```python
from build123d import *

# Parameters (mm, degrees)
F1_DEPTH = 10
F2_DEPTH = 12
F3_SIZE  = 5
F4_SIZE  = 1.99999
F5_R     = 10
F6_DEPTH = 5
F7_R     = 4.99999
F9_DEPTH = 3


# Not quite as in the source:
# - a fillet or chamfer is up to 0.001 mm smaller than in the source, because OpenCascade refuses the exact size


with BuildPart() as f1:
    # F0 (on Right) → F1 (new body)
    with BuildSketch(Plane.YZ):
        with BuildLine():
            Line((15, 5), (27.0370116692, 13))
            ThreePointArc((27.0370116692, 13), (21.2132034356, 21.2132034356), (13, 27.0370116692))
            Line((13, 27.0370116692), (5, 15))
            Line((5, 15), (0, 15))
            Line((0, 15), (-5, 15))
            Line((-5, 15), (-13, 27.0370116692))
            ThreePointArc((-13, 27.0370116692), (-21.2132034356, 21.2132034356), (-27.0370116692, 13))
            Line((-27.0370116692, 13), (-15, 5))
            Line((-15, 5), (-15, 0))
            Line((-15, 0), (-15, -5))
            Line((-15, -5), (-27.0370116692, -13))
            ThreePointArc((-27.0370116692, -13), (-21.2132034356, -21.2132034356), (-13, -27.0370116692))
            Line((-13, -27.0370116692), (-5, -15))
            Line((-5, -15), (0, -15))
            Line((0, -15), (5, -15))
            Line((5, -15), (13, -27.0370116692))
            ThreePointArc((13, -27.0370116692), (21.2132034356, -21.2132034356), (27.0370116692, -13))
            Line((27.0370116692, -13), (15, -5))
            Line((15, -5), (15, 0))
            Line((15, 0), (15, 5))
        make_face()
    extrude(amount=F1_DEPTH)

    # F0 (on Right) → F2 (join)
    with BuildSketch(Plane.YZ):
        with BuildLine():
            ThreePointArc((27.0370116692, -13), (29.2498747867, -6.6666952054), (30, 0))
            ThreePointArc((30, 0), (29.2498747867, 6.6666952054), (27.0370116692, 13))
            Line((27.0370116692, 13), (15, 5))
            Line((15, 5), (15, 0))
            Line((15, 0), (15, -5))
            Line((15, -5), (27.0370116692, -13))
        make_face()
        with BuildLine():
            ThreePointArc((27.0370116692, 13), (29.2498747867, 6.6666952054), (30, 0))
            ThreePointArc((30, 0), (29.2498747867, -6.6666952054), (27.0370116692, -13))
            Line((27.0370116692, -13), (34, -8))
            Line((34, -8), (34, 0))
            Line((34, 0), (34, 8))
            Line((34, 8), (27.0370116692, 13))
        make_face()
        with BuildLine():
            Line((5, 15), (13, 27.0370116692))
            ThreePointArc((13, 27.0370116692), (0, 30), (-13, 27.0370116692))
            Line((-13, 27.0370116692), (-5, 15))
            Line((-5, 15), (0, 15))
            Line((0, 15), (5, 15))
        make_face()
        with BuildLine():
            ThreePointArc((-13, 27.0370116692), (0, 30), (13, 27.0370116692))
            Line((13, 27.0370116692), (8, 34))
            Line((8, 34), (0, 34))
            Line((0, 34), (-8, 34))
            Line((-8, 34), (-13, 27.0370116692))
        make_face()
        with BuildLine():
            Line((-15, 5), (-27.0370116692, 13))
            ThreePointArc((-27.0370116692, 13), (-30, 0), (-27.0370116692, -13))
            Line((-27.0370116692, -13), (-15, -5))
            Line((-15, -5), (-15, 0))
            Line((-15, 0), (-15, 5))
        make_face()
        with BuildLine():
            ThreePointArc((-27.0370116692, -13), (-30, 0), (-27.0370116692, 13))
            Line((-27.0370116692, 13), (-34, 8))
            Line((-34, 8), (-34, 0))
            Line((-34, 0), (-34, -8))
            Line((-34, -8), (-27.0370116692, -13))
        make_face()
        with BuildLine():
            ThreePointArc((-13, -27.0370116692), (0, -30), (13, -27.0370116692))
            Line((13, -27.0370116692), (5, -15))
            Line((5, -15), (0, -15))
            Line((0, -15), (-5, -15))
            Line((-5, -15), (-13, -27.0370116692))
        make_face()
        with BuildLine():
            Line((8, -34), (13, -27.0370116692))
            ThreePointArc((13, -27.0370116692), (0, -30), (-13, -27.0370116692))
            Line((-13, -27.0370116692), (-8, -34))
            Line((-8, -34), (0, -34))
            Line((0, -34), (8, -34))
        make_face()
    extrude(amount=F2_DEPTH)

    # F3
    f3_edges = [f1.edges().sort_by_distance(p)[0] for p in [
        (10, 21.213203, 21.213203),
        (10, -21.213203, 21.213203),
        (10, -21.213203, -21.213203),
        (10, 21.213203, -21.213203),
    ]]
    chamfer(f3_edges, length=F3_SIZE)

    # F4 (size 2 in the source; OpenCascade refuses exactly that, so slightly less here)
    f4_edges = [f1.edges().sort_by_distance(p)[0] for p in [
        (12, 0, 34),
        (12, -10.5, 30.518506),
        (12, 10.5, 30.518506),
        (12, -9, 21.018506),
        (12, 9, 21.018506),
        (12, 0, 15),
        (12, -15, 0),
        (12, -21.018506, 9),
        (12, -30.518506, 10.5),
        (12, -34, 0),
        (12, -30.518506, -10.5),
        (12, -21.018506, -9),
        (12, 0, -15),
        (12, -9, -21.018506),
        (12, -10.5, -30.518506),
        (12, 0, -34),
        (12, 10.5, -30.518506),
        (12, 9, -21.018506),
        (12, 15, 0),
        (12, 21.018506, 9),
        (12, 30.518506, 10.5),
        (12, 34, 0),
        (12, 21.018506, -9),
        (12, 30.518506, -10.5),
    ]]
    chamfer(f4_edges, length=F4_SIZE)

    # F5 (on face) → F6 (join)
    with BuildSketch(Plane.YZ.offset(10)):
        Circle(F5_R)
    extrude(amount=F6_DEPTH)

    # F7 (radius 5 in the source; OpenCascade refuses exactly that, so slightly less here)
    f7_edges = [f1.edges().sort_by_distance(p)[0] for p in [
        (15, -10, 0),
    ]]
    fillet(f7_edges, radius=F7_R)

    # F8 (on face) → F9 (cut)
    with BuildSketch(Plane.YZ):
        with BuildLine():
            ThreePointArc((0, -15), (10.6066017178, -10.6066017178), (15, 0))
            ThreePointArc((15, 0), (10.6066017178, 10.6066017178), (0, 15))
            ThreePointArc((0, 15), (-10.6066017178, 10.6066017178), (-15, 0))
            ThreePointArc((-15, 0), (-10.6066017178, -10.6066017178), (0, -15))
        make_face()
    extrude(amount=F9_DEPTH, mode=Mode.SUBTRACT)


solid = f1.part
```
Model file for the job. Use its own axes, mm. A direction names the side the tool comes from. Give positions to 0.01 mm unless a question says otherwise; leave off trailing zeros. Write each loop counter-clockwise with the first axis right and the second up, starting at its lowest first coordinate (ties: lowest second). Pieces come first, ordered by that corner, then holes. Notation, with made-up numbers: M 16.5,32 L 28.5,32 A13 ccw 28.5,42 Z; hole C -31.5,70 d1. An arc over 180 degrees is marked long. Use a Markdown table: item, result.
1) Drill centre lines: line 1 (Z direction, x = 2.45, y = 0); line 2 (Y direction, x = 8.25, z = 12.5); line 3 (X direction, y = 3, z = 24.5). Where is each one in solid material? Low to high. Write a range as from..to.
Responses:
| item | result |
|---|---|
| line 1 | z = -34..-15, 15..34 |
| line 2 | y = -27.73..-26.28, -23.65..23.65, 26.28..27.73 |
| line 3 | x = 0..12 |
2) Cut at D-D (x = 13.5). List the corners of the cut face in (y, z), and give its area (3 significant figures).
Responses:
| item | result |
|---|---|
| outline | C 0,0 d17.14 |
| area | 231 mm2 |
3) Pull direction Y, two halves, no side cores. Call faces 1 (the flat face through (8.41, 11.98, -25.5)), 2 (the flat face through (3, 0, 0)), 3 (the flat face through (11.014, -8.212, 21.664)), 4 (the flat face through (11.014, -21.664, -8.212)): +Y half, -Y half, draft (parallel to the pull), parting line (faces both ways), or undercut.
Responses:
| item | result |
|---|---|
| face 1 | +Y half |
| face 2 | undercut |
| face 3 | -Y half |
| face 4 | undercut |
4) Tool access for faces 5 (the flat face through (10, 10, -5)), 6 (the flat face through (11, 0, 16)), 7 (the flat face through (12, 0, 25)), 8 (the flat face through (8.41, -11.98, 25.5)): list every direction of +Z, -Z, +X, -X, +Y, -Y with a clear straight run to the whole face (end or side of a thin tool).
Responses:
| item | result |
|---|---|
| face 5 | +X |
| face 6 | +X, +Y, -Y |
| face 7 | +Z, +X, +Y, -Y |
| face 8 | +X, -Y |
5) Cut at C-C (x = 7.75). List the corners of the cut face in (y, z), and give its area (3 significant figures).
Responses:
| item | result |
|---|---|
| outline | M -34,-8 L -27.04,-13 L -24.72,-11.46 A27.25 ccw -11.46,-24.72 L -13,-27.04 L -8,-34 L 8,-34 L 13,-27.04 L 11.46,-24.72 A27.25 ccw 24.72,-11.46 L 27.04,-13 L 34,-8 L 34,8 L 27.04,13 L 24.72,11.46 A27.25 ccw 11.46,24.72 L 13,27.04 L 8,34 L -8,34 L -13,27.04 L -11.46,24.72 A27.25 ccw -24.72,11.46 L -27.04,13 L -34,8 Z |
| area | 2,990 mm2 |
6) Pin check, flat tips, straight feed: pin 1 (3 mm diameter, centred on x = 6, y = -18.5, fed in from -Z); pin 2 (3 mm diameter, centred on x = 8, z = -19, fed in from +Y); pin 3 (16.5 mm diameter, centred on y = 27.5, z = -1, fed in from +X). Stop position of each tip, or through.
Responses:
| item | result |
|---|---|
| pin 1 | stops at z = -24.45 |
| pin 2 | stops at y = 21.63 |
| pin 3 | stops at x = 12 |
